```python
from build123d import *

# Parameters (mm, degrees)
SKETCH1_W           = 25
SKETCH1_H           = 15
BOSS_EXTRUDE1_DEPTH = 1.3
BOSS_EXTRUDE2_DEPTH = 0.1
SKETCH3_W           = 4.723765288
SKETCH3_H           = 5
SKETCH3_W_2         = 2.5
SKETCH3_H_2         = 4.03488285
BOSS_EXTRUDE3_DEPTH = 1


with BuildPart() as part:
    # Sketch1 → Boss-Extrude1 (new body)
    with BuildSketch(Plane(origin=(0, 0, 0), x_dir=(1, 0, 0), z_dir=(0, 1, 0))):
        Rectangle(SKETCH1_W, SKETCH1_H)
    extrude(amount=BOSS_EXTRUDE1_DEPTH)

    # Sketch2 → Boss-Extrude2 (add)
    with BuildSketch(Plane(origin=(0, 1.3, 0), x_dir=(1, 0, 0), z_dir=(0, 1, 0))):
        Polygon((-3.654721125, -5.569339468), (-12.030839718, -5.569339468), (-12.030839718, -3.469339468), (-7.030839718, -3.469339468), (-7.030839718, -2.769339468), (-12.071748872, -2.769339468), (-12.071748872, -0.669339468), (-7.060469733, -0.669339468), (-7.060469733, 0.030660532), (-12.030839718, 0.030660532), (-12.030839718, 2.130660532), (-7.030839718, 2.130660532), (-7.030839718, 2.830660532), (-12.030839718, 2.830660532), (-12.030839718, 6.830660532), (-11.330839718, 6.830660532), (-11.330839718, 3.530660532), (-6.330839718, 3.530660532), (-6.330839718, 1.430660532), (-11.330839718, 1.430660532), (-11.330839718, 0.730660532), (-6.360469733, 0.730660532), (-6.360469733, -1.369339468), (-11.360469733, -1.369339468), (-11.360469733, -2.069339468), (-6.330839718, -2.069339468), (-6.330839718, -4.169339468), (-11.330839718, -4.169339468), (-11.330839718, -4.869339468), (-4.354721125, -4.869339468), (-4.354721125, 2.346150012), (-3.654721125, 2.346150012), align=None)
    extrude(amount=BOSS_EXTRUDE2_DEPTH)

    # Sketch3 → Boss-Extrude3 (add)
    with BuildSketch(Plane(origin=(0, 1.3, 0), x_dir=(1, 0, 0), z_dir=(0, 1, 0))):
        with Locations((0.147617665, 1.651198425)):
            Rectangle(SKETCH3_W, SKETCH3_H)
        with Locations((1.259500309, -3.727346048)):
            Rectangle(SKETCH3_W_2, SKETCH3_H_2)
    extrude(amount=BOSS_EXTRUDE3_DEPTH)


solid = part.part
```
CAD build for the part. Positions are in the model's coordinates, mm. A direction names the side the tool comes from. Give positions to 0.01 mm unless a question says otherwise; leave off trailing zeros. Order: outer loops, then holes, each group sorted by start corner. A loop starts at its lowest first (then second) coordinate and runs counter-clockwise, first axis right, second up.
(1) Tool access for faces 4 (the flat face through (1, 2, 5.745)), 5 (the flat face through (2.51, 2, 4)), 6 (the flat face through (1, 2.3, 4)): list every direction of +Z, -Z, +X, -X, +Y, -Y with a clear straight run to the whole face (end or side of a thin tool).
(2) Mould opens along Z. For faces 1 (the flat face through (1, 2, 1.71)), 2 (the flat face through (0, 1, -7.5)), 3 (the flat face through (-2.214, 2, -2)) say: released by +Z, released by -Z, zero draft, split by the parting line, or undercut.
(3) Flat gauge pins, fed straight in: pin 1 (0.8 mm diameter, centred on y = 2, z = -1, fed in from -X); pin 2 (4.5 mm diameter, centred on x = 5, z = -1, fed in from +Y); pin 3 (1.1 mm diameter, centred on x = 0, y = 2, fed in from -Z). Where does each tip first touch, or does it go through?
(4) Drill centre lines: L1, parallel to X at y = 1.35, z = 1; L2, parallel to Y at x = -9, z = 0; L3, parallel to X at y = 1.85, z = 1.75. Where is each one in solid material? Low to high.
(5) Saw through at C-C, the plane z = -1.75. Give the cut face in (x, y).
(6) Saw through at B-B, the plane x = -4. Give the cut face in (y, z).
(7) Saw through at A-A, the plane y = 1.7. Give the cut face in (x, z), then the cut area to 3 significant figures.
(8) Saw through at D-D, the plane z = 0.25. Give the cut face in (x, y), then the cut area to 3 significant figures.
Results found:
1. face 4: +Z, +X, -X, +Y
1. face 5: +Z, -Z, +X, +Y
1. face 6: +Z, -Z, +X, -X, +Y
2. face 1: undercut
2. face 2: released by -Z
2. face 3: zero draft
3. pin 1: stops at x = -2.21
3. pin 2: stops at y = 1.3
3. pin 3: stops at z = -4.15
4. L1: x = -12.07 to -6.36, -4.35 to -3.65
4. L2: y = 0 to 1.3
4. L3: x = 0.01 to 2.51
5. outline: (-12.5, 0) - (12.5, 0) - (12.5, 1.3) - (2.51, 1.3) - (2.51, 2.3) - (-2.21, 2.3) - (-2.21, 1.3) - (-3.65, 1.3) - (-3.65, 1.4) - (-4.35, 1.4) - (-4.35, 1.3) - (-6.33, 1.3) - (-6.33, 1.4) - (-12.03, 1.4) - (-12.03, 1.3) - (-12.5, 1.3) - close
6. outline: (0, -7.5) - (1.3, -7.5) - (1.3, -2.35) - (1.4, -2.35) - (1.4, 5.57) - (1.3, 5.57) - (1.3, 7.5) - (0, 7.5) - close
7. outline: (-2.21, -4.15) - (2.51, -4.15) - (2.51, 0.85) - (-2.21, 0.85) - close; (0.01, 1.71) - (2.51, 1.71) - (2.51, 5.74) - (0.01, 5.74) - close
7. area: 33.7 mm2
8. outline: (-12.5, 0) - (12.5, 0) - (12.5, 1.3) - (2.51, 1.3) - (2.51, 2.3) - (-2.21, 2.3) - (-2.21, 1.3) - (-3.65, 1.3) - (-3.65, 1.4) - (-4.35, 1.4) - (-4.35, 1.3) - (-6.36, 1.3) - (-6.36, 1.4) - (-7.06, 1.4) - (-7.06, 1.3) - (-12.5, 1.3) - close
8. area: 37.4 mm2
